The figure shows three views and two pictorial views of one solid part (mm, origin at its lowest corner). Answer the questions. Give positions to 0.01 mm unless a question says otherwise; leave off trailing zeros. Loops run counter-clockwise (first coordinate to the right, second up) from the corner with the lowest first, then second, coordinate; pieces in that order, holes last.
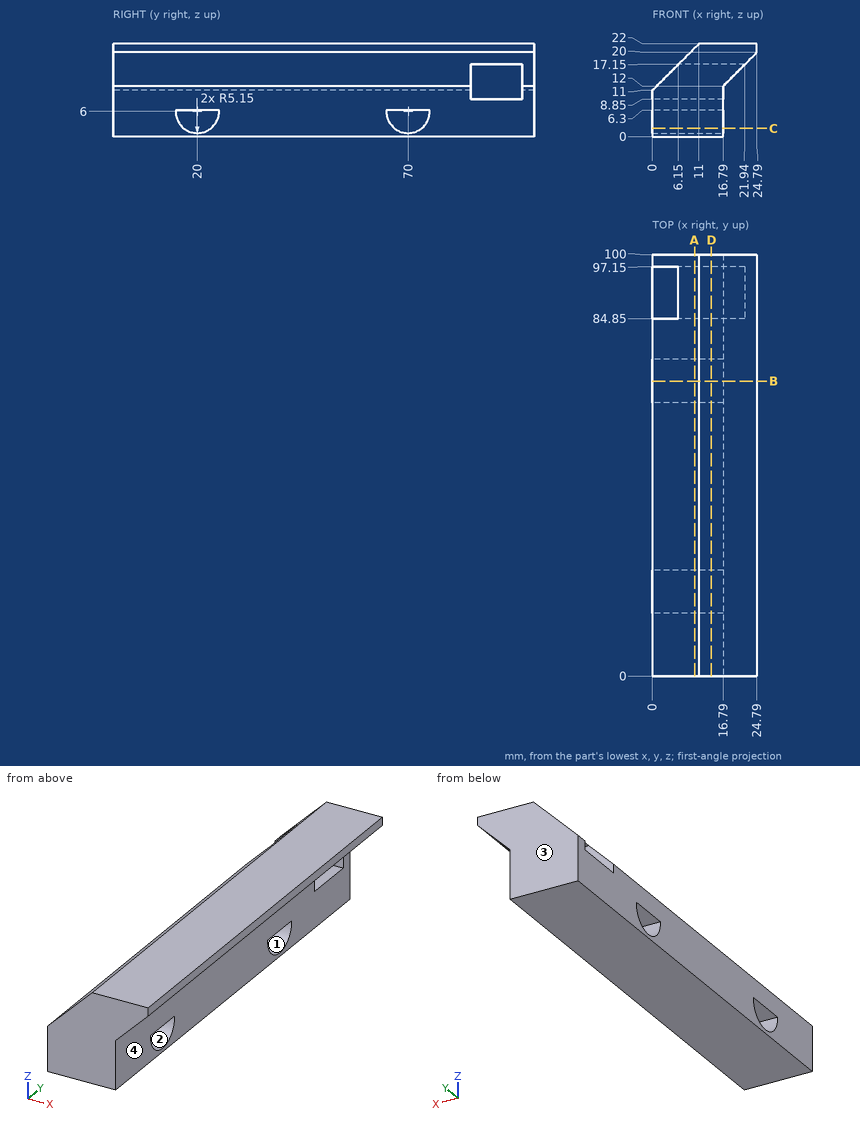
Q1. Consider line 1 along Y through (x, z) = (16, 15.5); line 2 along Z through (x, y) = (13, 87); line 3 along X through (y, z) = (34, 6). Determine where each line is inside the solid, lowest interval first.
Q2. Section C-C on z = 2 is taken. Give the vertices of the cut face in (x, y).
Q3. Determine the mould class of the marked faces 1, 2, 3 and 4 for opening direction Y: +Y half, -Y half, draft (parallel to the pull), parting line (faces both ways), or undercut.
Q4. Section D-D on x = 14 is taken. Give the vertices of the cut face in (y, z), plus the area to 3 significant figures.
Q5. Given pin 1 (3.5 mm diameter, centred on y = 32.5, z = 8.5, fed in from +X); pin 2 (6 mm diameter, centred on x = 20, z = 2.5, fed in from +Y); pin 3 (10 mm diameter, centred on y = 42.5, z = 14.5, fed in from +X), each flat-ended and moving along its own axis, determine where each tip first touches the part or whether it passes through.
Q6. Section B-B on y = 70 is taken. Give the vertices of the cut face in (x, z).
Q7. Section A-A on x = 10 is taken. Give the vertices of the cut face in (y, z), plus the area to 3 significant figures.
Check result:
1. line 1: y = 0 to 84.85, 97.15 to 100
1. line 2: z = 0 to 8.85, 17.15 to 22
1. line 3: x = 0 to 16.79
2. outline: (0, 0) - (16.79, 0) - (16.79, 16.76) - (0, 16.76) - close; (0, 23.24) - (16.79, 23.24) - (16.79, 66.76) - (0, 66.76) - close; (0, 73.24) - (16.79, 73.24) - (16.79, 100) - (0, 100) - close
3. face 1: undercut
3. face 2: undercut
3. face 3: +Y half
3. face 4: draft
4. outline: (0, 0) - (100, 0) - (100, 22) - (0, 22) - close; hole (14.86, 6.3) arc R5.15 ccw (long way) to (25.14, 6.3) - close; hole (64.86, 6.3) arc R5.15 ccw (long way) to (75.14, 6.3) - close; hole (84.85, 8.85) - (97.15, 8.85) - (97.15, 17.15) - (84.85, 17.15) - close
4. area: 2,010 mm2
5. pin 1: stops at x = 16.79
5. pin 2: passes through
5. pin 3: stops at x = 24.29
6. outline: (0, 0) - (16.79, 0) - (16.79, 0.85) - (0, 0.85) - close; (0, 6.3) - (16.79, 6.3) - (16.79, 12) - (24.79, 20) - (24.79, 22) - (11, 22) - (0, 11) - close
7. outline: (0, 0) - (100, 0) - (100, 21) - (0, 21) - close; hole (14.86, 6.3) arc R5.15 ccw (long way) to (25.14, 6.3) - close; hole (64.86, 6.3) arc R5.15 ccw (long way) to (75.14, 6.3) - close; hole (84.85, 8.85) - (97.15, 8.85) - (97.15, 17.15) - (84.85, 17.15) - close
7. area: 1,910 mm2
